from build123d import *

# Parameters (mm, degrees)
F0_W      = 42
F0_H      = 42
F1_DEPTH  = 42
F2_SIZE   = 2.5
F3_R      = 1.5
F4_DEPTH  = 10
F5_R      = 11
F6_DEPTH  = 2
F8_DEPTH  = 24
F9_W      = 15
F9_H      = 5
F10_DEPTH = 7.5


with BuildPart() as f1:
    # F0 (on Top) → F1 (new body)
    with BuildSketch(Plane.XY):
        Rectangle(F0_W, F0_H)
    extrude(amount=F1_DEPTH)

    # F2
    f2_edges = [f1.edges().sort_by_distance(p)[0] for p in [
        (-21, -21, 21),
        (21, -21, 21),
        (21, 21, 21),
        (-21, 21, 21),
    ]]
    chamfer(f2_edges, length=F2_SIZE)

    # F3 (on face) → F4 (cut)
    with BuildSketch(Plane.XY.offset(42)):
        with Locations((-15.5, 15.5)):
            Circle(F3_R)
        with Locations((15.5, 15.5)):
            Circle(F3_R)
        with Locations((15.5, -15.5)):
            Circle(F3_R)
        with Locations((-15.5, -15.5)):
            Circle(F3_R)
    extrude(amount=-F4_DEPTH, mode=Mode.SUBTRACT)

    # F5 (on face) → F6 (join)
    with BuildSketch(Plane.XY.offset(42)):
        Circle(F5_R)
    extrude(amount=F6_DEPTH)

    # F7 (on face) → F8 (join)
    with BuildSketch(Plane.XY.offset(44)):
        with BuildLine():
            Line((2.193171, 1.2), (-2.193171, 1.2))
            ThreePointArc((-2.193171, 1.2), (0, -2.5), (2.193171, 1.2))
        make_face()
    extrude(amount=F8_DEPTH)

    # F9 (on face) → F10 (join)
    with BuildSketch(Plane.XZ.offset(21)):
        with Locations((0, 7.5)):
            Rectangle(F9_W, F9_H)
    extrude(amount=F10_DEPTH)


solid = f1.part
Geometry: final body of the model. Coordinates: model frame, mm. A direction names the side the tool comes from. Round coordinates to 2 decimals unless told otherwise and drop trailing zeros. Loops run counter-clockwise (first coordinate to the right, second up) from the corner with the lowest first, then second, coordinate; pieces in that order, holes last. Notation, with made-up numbers: (58.25, 29) -> (98.25, 29) arc R29 cw to (98.25, 62) -> close; hole circle Ø5 at (23, -6). An arc over 180 degrees is marked (long way). One line per question, with ' | ' between items. Start each with the question number.
1. Line query: line 1 along Y through (x, z) = (-15.5, 38); line 2 along Y through (x, z) = (-15, 39). Output: solid intervals per line, ascending. Write a range as [from, to].
2. Section D-D on y = -8. Output: boundary loops of the cut face in (x, z), and give its area (3 significant figures).
3. Section B-B on y = 15.5. Output: boundary loops of the cut face in (x, z), and give its area (3 significant figures).
4. Contact query for flat-ended pins moving along their axis: pin 1 (1.5 mm diameter, centred on x = 15.5, y = 16, fed in from +Z); pin 2 (5 mm diameter, centred on x = -4.5, z = 29.5, fed in from -Y); pin 3 (2 mm diameter, centred on x = -5, y = 15, fed in from +Z). Output: stop coordinate, or through.
5. Mould query, pull axis X, two halves, no side actions, for faces 4 (the face through (0, -21, 21)), 5 (the face through (-17, 15.57, 37.07)), 6 (the face through (19.8, -19.7, 20.7)). Classes: pulls with the +X half, pulls with the -X half, needs draft (parallel to the pull), parting line crosses it, or undercut.
6. Set-up query: faces 1 (the face through (-0.1, -2.5, 55.8)), 2 (the face through (0, -25, 5)), 3 (the face through (0, 1.2, 56)). Return all of +Z, -Z, +X, -X, +Y, -Y with unobstructed straight access to the full face (end or side cutting, diameter ignored); none if empty.
7. Section A-A on x = 0. Output: boundary loops of the cut face in (y, z), and give its area (3 significant figures).
8. Section C-C on z = 8.5. Output: boundary loops of the cut face in (x, y).
Returned:
1) line 1: y = [-21, -17], [-14, 14], [17, 21] | line 2: y = [-21, -16.91], [-14.09, 14.09], [16.91, 21]
2) outline: (-21, 0) -> (21, 0) -> (21, 42) -> (7.55, 42) -> (7.55, 44) -> (-7.55, 44) -> (-7.55, 42) -> (-21, 42) -> close | area: 1,790 mm2
3) outline: (-21, 0) -> (21, 0) -> (21, 42) -> (17, 42) -> (17, 32) -> (14, 32) -> (14, 42) -> (-14, 42) -> (-14, 32) -> (-17, 32) -> (-17, 42) -> (-21, 42) -> close | area: 1,700 mm2
4) pin 1: stops at z = 32 | pin 2: stops at y = -21 | pin 3: stops at z = 42
5) face 4: needs draft | face 5: undercut | face 6: pulls with the +X half
6) face 1: +Z | face 2: -Z, +X, -X, -Y | face 3: +Z, +X, -X, +Y
7) outline: (-28.5, 5) -> (-21, 5) -> (-21, 0) -> (21, 0) -> (21, 42) -> (11, 42) -> (11, 44) -> (1.2, 44) -> (1.2, 68) -> (-2.5, 68) -> (-2.5, 44) -> (-11, 44) -> (-11, 42) -> (-21, 42) -> (-21, 10) -> (-28.5, 10) -> close | area: 1,930 mm2
8) outline: (-21, -18.5) -> (-18.5, -21) -> (-7.5, -21) -> (-7.5, -28.5) -> (7.5, -28.5) -> (7.5, -21) -> (18.5, -21) -> (21, -18.5) -> (21, 18.5) -> (18.5, 21) -> (-18.5, 21) -> (-21, 18.5) -> close
